Part model, mm, in its own coordinate system. Face numbers are marked on the shaded views. A direction names the side the tool comes from. Round coordinates to 2 decimals unless told otherwise and drop trailing zeros. Loops run counter-clockwise (first coordinate to the right, second up) from the corner with the lowest first, then second, coordinate; pieces in that order, holes last. Notation, with made-up numbers: M 49.25,-3.5 L 90.25,-3.5 A19 cw 90.25,19.5 Z; hole C 69,80.25 d3. An arc over 180 degrees is marked long. Answer as CSV lines item,"result". Start each with the question number.
Item 1: Drop flat-ended pins along their axis: pin 1 Ø8 at (y, z) = (36, 18.5) entering from +X; pin 2 Ø6 at (x, y) = (-11.5, 35) entering from +Z; pin 3 Ø5 at (x, y) = (11.5, 17.5) entering from +Z; pin 4 Ø12 at (x, z) = (-2, 12) entering from -Y. Give the stop position or say it passes through.
Item 2: Which spindle directions (+Z, -Z, +X, -X, +Y, -Y) get a long thin tool onto all of the face, cutting with end or side? Do the marked faces 4, 5 and 6. Say none if no direction does.
Item 3: Band-saw the part on A-A (z = 0). Give the cut face in (x, y), and give its area (3 significant figures).
Item 4: Wall check: line 1 (Y direction, x = -6, z = 39); line 2 (X direction, y = 19.5, z = 5); line 3 (X direction, y = 34, z = 1.5). Give the ranges that are in metal, low to high.
Item 5: Band-saw the part on C-C (y = 17.5). Give the cut face in (x, z), and give its area (3 significant figures).
Item 6: Mould opens along Z. For the marked faces 1, 2 and 3 say: pulls with the +Z half, pulls with the -Z half, needs draft (parallel to the pull), parting line crosses it, or undercut.
Item 7: Band-saw the part on B-B (x = 0). Give the cut face in (y, z), and give its area (3 significant figures).
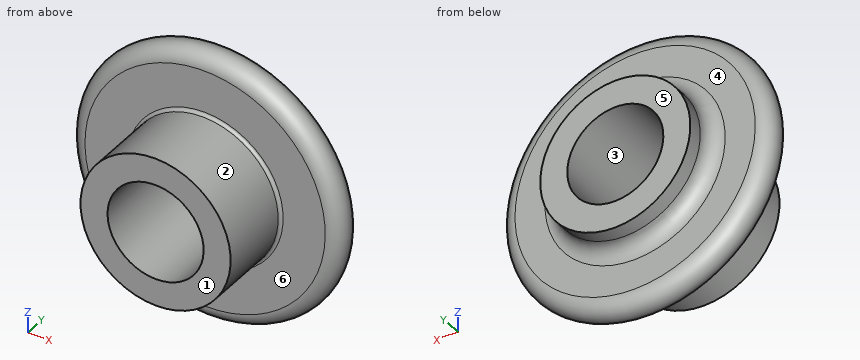
```python
from build123d import *

# Parameters (mm, degrees)
M36_TAPPED_HOLE1_D = 32
FILLET1_R          = 5
FILLET2_R          = 1


with BuildPart() as part:
    # Sketch1 → Revolve1 (revolve)
    with BuildSketch(Plane.XY, mode=Mode.PRIVATE) as revolve1_sk:
        with BuildLine():
            Line((0, 0), (0, 45))
            Line((0, 45), (25, 45))
            Line((25, 45), (25, 35))
            Line((25, 35), (40, 35))
            ThreePointArc((40, 35), (45, 30), (40, 25))
            Line((40, 25), (25, 25))
            Line((25, 25), (25, 0))
            Line((25, 0), (0, 0))
        make_face()
    revolve(revolve1_sk.sketch.rotate(Axis((0, 0, 0), (0, 1, 0)), 90), axis=Axis((0, 0, 0), (0, 1, 0)))

    # M36 Tapped Hole1 (through all)
    with Locations(Plane.ZX.offset(45)):
        with Locations((0, 0)):
            Hole(M36_TAPPED_HOLE1_D / 2)

    # Fillet1
    fillet1_edges = [part.edges().sort_by_distance(p)[0] for p in [
        (0, 35, 25),
    ]]
    fillet(fillet1_edges, radius=FILLET1_R)

    # Fillet2
    fillet2_edges = [part.edges().sort_by_distance(p)[0] for p in [
        (0, 25, 25),
    ]]
    fillet(fillet2_edges, radius=FILLET2_R)


solid = part.part
```
Answer block:
1,pin 1,"stops at x = 41.12"
1,pin 2,"stops at z = 43.26"
1,pin 3,"stops at z = 23.32"
1,pin 4,"stops at y = 0"
2,face 4,"+Y"
2,face 5,"+Z, -Z, +X, -X, +Y"
2,face 6,"-Y"
3,outline,"M -40,25 L -26,25 A1 cw -25,24 L -25,0 L -16,0 L -16,45 L -25,45 L -25,40 A5 cw -30,35 L -40,35 A5 ccw Z; M 16,0 L 25,0 L 25,24 A1 cw 26,25 L 40,25 A5 ccw 40,35 L 30,35 A5 cw 25,40 L 25,45 L 16,45 Z"
3,area,"1,200 mm^2"
4,line 1,"y = 25 to 35"
4,line 2,"x = -24.49 to -15.2, 15.2 to 24.49"
4,line 3,"x = -42.97 to -15.93, 15.93 to 42.97"
5,outline,"C 0,0 d50; hole C 0,0 d32"
5,area,"1,160 mm^2"
6,face 1,"needs draft"
6,face 2,"parting line crosses it"
6,face 3,"undercut"
7,outline,"M 0,-25 L 24,-25 A1 cw 25,-26 L 25,-40 A5 ccw 35,-40 L 35,-30 A5 cw 40,-25 L 45,-25 L 45,-16 L 0,-16 Z; M 0,16 L 45,16 L 45,25 L 40,25 A5 cw 35,30 L 35,40 A5 ccw 25,40 L 25,26 A1 cw 24,25 L 0,25 Z"
7,area,"1,200 mm^2"
